Can you work these out from the model? Positions are in its coordinate system, mm. A direction names the side the tool comes from. Give positions to 0.01 mm unless a question says otherwise; leave off trailing zeros. Loops run counter-clockwise (first coordinate to the right, second up) from the corner with the lowest first, then second, coordinate; pieces in that order, holes last. Notation, with made-up numbers: (50, 38) -> (106, 38) arc R11 cw to (106, 59) -> close; hole circle Ø5 at (27.5, -31). An arc over 180 degrees is marked (long way). One line per question, with ' | ' between items.
from build123d import *

# Parameters (mm, degrees)
SKETCH1_R                = 14
SKETCH1_R_2              = 1
SKETCH1_R_3              = 3
BOSS_EXTRUDE1_DEPTH      = 3
BOSS_EXTRUDE2_DEPTH      = 15
BOSS_EXTRUDE2_DEPTH_BACK = 1
SKETCH2_R                = 16
SKETCH2_R_2              = 14
SKETCH3_R                = 8.05
BOSS_EXTRUDE3_DEPTH      = 4
CUT_EXTRUDE1_DEPTH       = 10
CUT_EXTRUDE1_DEPTH_BACK  = 30
SKETCH4_R                = 2.5
SKETCH5_R                = 1.5
CUT_EXTRUDE2_DEPTH       = 37.483814873


with BuildPart() as part:
    # Sketch1 → Boss-Extrude1 (new body)
    # profile 1 of 2: a face of its own
    with BuildSketch(Plane.XY):
        Circle(SKETCH1_R)
        with Locations((0, -8)):
            Circle(SKETCH1_R_2, mode=Mode.SUBTRACT)
        with BuildLine():
            ThreePointArc((7.247844507, -5.126524164), (7.247844507, -7.247844507), (5.126524164, -7.247844507))
            Line((5.126524164, -7.247844507), (0.776457135, -2.897777479))
            ThreePointArc((0.776457135, -2.897777479), (0, -3), (-0.776457135, -2.897777479))
            Line((-0.776457135, -2.897777479), (-5.126524164, -7.247844507))
            ThreePointArc((-5.126524164, -7.247844507), (-7.247844507, -7.247844507), (-7.247844507, -5.126524164))
            Line((-7.247844507, -5.126524164), (-2.897777479, -0.776457135))
            ThreePointArc((-2.897777479, -0.776457135), (-3, 0), (-2.897777479, 0.776457135))
            Line((-2.897777479, 0.776457135), (-7.247844507, 5.126524164))
            ThreePointArc((-7.247844507, 5.126524164), (-7.247844507, 7.247844507), (-5.126524164, 7.247844507))
            Line((-5.126524164, 7.247844507), (-0.776457135, 2.897777479))
            ThreePointArc((-0.776457135, 2.897777479), (0, 3), (0.776457135, 2.897777479))
            Line((0.776457135, 2.897777479), (5.126524164, 7.247844507))
            ThreePointArc((5.126524164, 7.247844507), (7.247844507, 7.247844507), (7.247844507, 5.126524164))
            Line((7.247844507, 5.126524164), (2.897777479, 0.776457135))
            ThreePointArc((2.897777479, 0.776457135), (2.974334584, 0.391578577), (3, 0))
            ThreePointArc((3, 0), (2.974334584, -0.391578577), (2.897777479, -0.776457135))
            Line((2.897777479, -0.776457135), (7.247844507, -5.126524164))
        make_face(mode=Mode.SUBTRACT)
        with Locations((-9.5, 0)):
            Circle(SKETCH1_R_2, mode=Mode.SUBTRACT)
        with Locations((9.5, 0)):
            Circle(SKETCH1_R_2, mode=Mode.SUBTRACT)
        with Locations((0, 8)):
            Circle(SKETCH1_R_2, mode=Mode.SUBTRACT)
    # profile 2 of 2: a face of its own
    with BuildSketch(Plane.XY):
        Circle(SKETCH1_R_3)
    extrude(amount=BOSS_EXTRUDE1_DEPTH)

    # Sketch2 → Boss-Extrude2 (add, two sides: drawn at the far end of the back side and taken through both)
    with BuildSketch(Plane.XY.offset(3).offset(-BOSS_EXTRUDE2_DEPTH_BACK)):
        Circle(SKETCH2_R)
        Circle(SKETCH2_R_2, mode=Mode.SUBTRACT)
    extrude(amount=BOSS_EXTRUDE2_DEPTH + BOSS_EXTRUDE2_DEPTH_BACK)

    # Sketch3 → Boss-Extrude3 (add, symmetric)
    with BuildSketch(Plane(origin=(0, 0, 0), x_dir=(0.7071067811865477, 0.7071067811865475, 0), z_dir=(-0.7071067811865475, 0.7071067811865477, 0))):
        with BuildLine():
            Line((-9.05, 9.05), (-9.05, 0))
            Line((-9.05, 0), (9.05, 0))
            Line((9.05, 0), (9.05, 9.05))
            Line((9.05, 9.05), (9.05, 12.166022099))
            ThreePointArc((9.05, 12.166022099), (8.879286309, 12.974546435), (8.396288399, 13.645044596))
            Line((8.396288399, 13.645044596), (6.091955006, 15.742576798))
            ThreePointArc((6.091955006, 15.742576798), (0, 18.1), (-6.091955006, 15.742576798))
            Line((-6.091955006, 15.742576798), (-8.396288399, 13.645044596))
            ThreePointArc((-8.396288399, 13.645044596), (-8.879286309, 12.974546435), (-9.05, 12.166022099))
            Line((-9.05, 12.166022099), (-9.05, 9.05))
        make_face()
        with Locations(Location((0, 9.05, 0), (0, 0, 180))):
            Circle(SKETCH3_R, mode=Mode.SUBTRACT)
    extrude(amount=BOSS_EXTRUDE3_DEPTH, both=True)

    # Sketch4 → Cut-Extrude1 (cut, two sides: drawn at the far end of the back side and taken through both)
    with BuildSketch(Plane(origin=(0, 0, 0), x_dir=(-1, 0, 0), z_dir=(0, 0, -1)).offset(-CUT_EXTRUDE1_DEPTH_BACK)):
        with Locations(Location((0, 0, 0), (0, 0, 180))):
            Circle(SKETCH4_R)
    extrude(amount=CUT_EXTRUDE1_DEPTH + CUT_EXTRUDE1_DEPTH_BACK, mode=Mode.SUBTRACT)

    # Sketch5 → Cut-Extrude2 (cut, through all)
    with BuildSketch(Plane(origin=(6.39931637, 6.39931637, 0), x_dir=(0, 0, -1), z_dir=(0.7071067811865476, 0.7071067811865476, 0))):
        with Locations(Location((9.05, 0, 0), (0, 0, 90))):
            Circle(SKETCH5_R)
    extrude(amount=-CUT_EXTRUDE2_DEPTH, mode=Mode.SUBTRACT)


solid = part.part
Q1. On a 3-axis mill with a long thin cutter (end or side, diameter ignored), from which of +Z, -Z, +X, -X, +Y, -Y can I reach the whole of each face in a straight line? I mean faces 1 (the face through (-2.59, -2.67, -16.19)), 2 (the face through (-3.47, -15.62, 9.89)), 3 (the face through (12.932, -5.362, 0.986)), 4 (the face through (0, -3, 3)), 5 (the face through (-4.28, 1.376, -1.048)). Say none if no direction works.
Entries:
face 1: none | face 2: +Z, -Z | face 3: -Z | face 4: +Z | face 5: -Z, -X, +Y
Q2. If we section it at A-A (z = -7): Write out the boundary of the cut face in (x, y).
Entries:
outline: (-9.23, -3.57) -> (-3.57, -9.23) -> (-2.68, -8.33) -> (-8.33, -2.68) -> close; (2.68, 8.33) -> (8.33, 2.68) -> (9.23, 3.57) -> (3.57, 9.23) -> close
Q3. If I drill on probe 1 along Y at (x, z) = (0, 1); probe 2 along Y at (x, z) = (0, 16); probe 3 along Z at (x, y) = (-5, 2), over which ranges is the centre line in solid material (lowest first)? Write a range as from..to.
Entries:
probe 1: -14..-9, -7..-2.5, 2.5..7, 9..14 | probe 2: -16..-14, 14..16 | probe 3: 0..3
Q4. If we section it at D-D (x = -11.5): Write out the boundary of the cut face in (y, z), plus the area to 3 significant figures.
Entries:
outline: (-11.12, 2) -> (-7.98, 2) -> (-7.98, 0) -> (7.98, 0) -> (7.98, 2) -> (11.12, 2) -> (11.12, 18) -> (7.98, 18) -> (7.98, 3) -> (-7.98, 3) -> (-7.98, 18) -> (-11.12, 18) -> close | area: 148 mm²
Q5. If we section it at C-C (z = 15): Write out the boundary of the cut face in (x, y), plus the area to 3 significant figures.
Entries:
outline: circle Ø32 at (0, 0); hole circle Ø28 at (0, 0) | area: 188 mm²
Q6. If we section it at B-B (y = 10): Write out the boundary of the cut face in (x, z), plus the area to 3 significant figures.
Entries:
outline: (-12.49, 2) -> (-9.8, 2) -> (-9.8, 0) -> (9.8, 0) -> (9.8, 2) -> (12.49, 2) -> (12.49, 18) -> (9.8, 18) -> (9.8, 3) -> (-9.8, 3) -> (-9.8, 18) -> (-12.49, 18) -> close | area: 145 mm²
Q7. For pin 1 Ø1 at (x, z) = (-8, -6) entering from +Y; pin 2 Ø12 at (x, y) = (-11, 9.5) entering from -Z; pin 3 Ø4 at (x, y) = (0, 0) entering from +Z; pin 4 Ø1.6 at (x, y) = (-9.5, 0) entering from -Z, each with a flat end and sliding along its axis, tell me the tip position at first contact or that it passes through.
Entries:
pin 1: y = -2.28 | pin 2: z = 0 | pin 3: z = -16.85 | pin 4: through
Q8. If we mould it in two halves opening along X, with no side actions, what happens to faces 6 (the face through (4, 4, 0)), 7 (the face through (-6.4, -6.4, -6.2)), 8 (the face through (0, -6, 0)), 9 (the face through (5.04, -2.92, 1.48))? For each: pulls with the +X half, pulls with the -X half, needs draft (parallel to the pull), parting line crosses it, or undercut.
Entries:
face 6: undercut | face 7: pulls with the -X half | face 8: needs draft | face 9: undercut
